Can you work these out from the model? Positions are in its coordinate system, mm. A direction names the side the tool comes from. Round coordinates to 2 decimals unless told otherwise and drop trailing zeros. Loops run counter-clockwise (first coordinate to the right, second up) from the corner with the lowest first, then second, coordinate; pieces in that order, holes last. Notation, with made-up numbers: (60, 49.25) -> (96, 49.25) arc R16 ccw to (96, 53.25) -> close; hole circle Ø6 at (63.5, -26.5). An arc over 180 degrees is marked (long way). Write item = value, one per line.
from build123d import *

# Parameters (mm, degrees)
SKETCH1_R           = 1.6
BOSS_EXTRUDE1_DEPTH = 7.2
SKETCH2_R           = 3.75
CUT_EXTRUDE1_DEPTH  = 5.7
CUT_EXTRUDE2_DEPTH  = 7.5
SKETCH5_W           = 7.75
SKETCH5_H           = 8.9
SKETCH5_W_2         = 9.25
BOSS_EXTRUDE2_DEPTH = 14.4
SKETCH6_W           = 10.1
SKETCH6_H           = 8.4
CUT_EXTRUDE3_DEPTH  = 4.5
FILLET1_R           = 1.75
FILLET2_R           = 1
CHAMFER1_SIZE       = 1.75
CUT_EXTRUDE4_DEPTH  = 3.3
CUT_EXTRUDE5_REACH  = 20.3
SKETCH8_W           = 10.1
SKETCH8_H           = 0.75
SKETCH9_W           = 10.1
SKETCH9_H           = 1.2
BOSS_EXTRUDE3_DEPTH = 5.5


with BuildPart() as part:
    # Sketch1 → Boss-Extrude1 (new body)
    with BuildSketch(Plane.XY):
        with BuildLine():
            ThreePointArc((18.5, 3.75), (22.25, 0), (18.5, -3.75))
            Line((18.5, -3.75), (14.75, -3.75))
            Line((14.75, -3.75), (14.75, -6.5))
            Line((14.75, -6.5), (-14.75, -6.5))
            Line((-14.75, -6.5), (-14.75, -3.75))
            Line((-14.75, -3.75), (-18.5, -3.75))
            ThreePointArc((-18.5, -3.75), (-22.25, 0), (-18.5, 3.75))
            Line((-18.5, 3.75), (-14.75, 3.75))
            Line((-14.75, 3.75), (-14.75, 6.5))
            Line((-14.75, 6.5), (14.75, 6.5))
            Line((14.75, 6.5), (14.75, 3.75))
            Line((14.75, 3.75), (18.5, 3.75))
        make_face()
        with Locations((-18.5, 0)):
            Circle(SKETCH1_R, mode=Mode.SUBTRACT)
        with Locations((18.5, 0)):
            Circle(SKETCH1_R, mode=Mode.SUBTRACT)
    extrude(amount=BOSS_EXTRUDE1_DEPTH)

    # Sketch2 → Cut-Extrude1 (cut)
    with BuildSketch(Plane.XY.offset(7.2)):
        with Locations((-18.5, 0)):
            Circle(SKETCH2_R)
        with Locations((18.5, 0)):
            Circle(SKETCH2_R)
    extrude(amount=-CUT_EXTRUDE1_DEPTH, mode=Mode.SUBTRACT)

    # Sketch4 → Cut-Extrude2 (cut)
    with BuildSketch(Plane.XZ.offset(3.75)):
        Polygon((-18.5, 1.5), (-16.95, 1.5), (-16.95, 3.5), (-14.75, 5.7), (-14.75, 7.2), (-18.5, 7.2), align=None)
        Polygon((18.5, 1.5), (16.95, 1.5), (16.95, 3.5), (14.75, 5.7), (14.75, 7.2), (18.5, 7.2), align=None)
    extrude(amount=-CUT_EXTRUDE2_DEPTH, mode=Mode.SUBTRACT)

    # Sketch5 → Boss-Extrude2 (add)
    with BuildSketch(Plane.XY.offset(7.2)):
        Polygon((-5.8, -5.95), (-14.75, -5.95), (-14.75, 5.95), (-5.8, 5.95), (-5.8, 4.2), (0, 4.2), (4.3, 4.2), (4.3, 5.95), (14.75, 5.95), (14.75, -5.95), (4.3, -5.95), (4.3, -4.2), (0, -4.2), (-5.8, -4.2), align=None)
        with Locations((-10.275, 0)):
            Rectangle(SKETCH5_W, SKETCH5_H, mode=Mode.SUBTRACT)
        with Locations((9.525, 0)):
            Rectangle(SKETCH5_W_2, SKETCH5_H, mode=Mode.SUBTRACT)
    extrude(amount=BOSS_EXTRUDE2_DEPTH)

    # Sketch6 → Cut-Extrude3 (cut)
    with BuildSketch(Plane.XY.offset(21.6)):
        with Locations((-0.75, 0)):
            Rectangle(SKETCH6_W, SKETCH6_H)
    extrude(amount=-CUT_EXTRUDE3_DEPTH, mode=Mode.SUBTRACT)

    # Fillet1
    fillet1_edges = [part.edges().sort_by_distance(p)[0] for p in [
        (4.3, 5.95, 14.4),
        (14.75, 5.95, 14.4),
        (14.75, -5.95, 14.4),
        (4.3, -5.95, 14.4),
        (-5.8, 5.95, 14.4),
        (-14.75, 5.95, 14.4),
        (-14.75, -5.95, 14.4),
        (-5.8, -5.95, 14.4),
    ]]
    fillet(fillet1_edges, radius=FILLET1_R)

    # Fillet2
    fillet2_edges = [part.edges().sort_by_distance(p)[0] for p in [
        (-6.4, 4.45, 14.4),
        (-14.15, 4.45, 14.4),
        (-14.15, -4.45, 14.4),
        (-6.4, -4.45, 14.4),
    ]]
    fillet(fillet2_edges, radius=FILLET2_R)

    # Chamfer1
    chamfer1_edges = [part.edges().sort_by_distance(p)[0] for p in [
        (14.15, 4.45, 14.4),
        (4.9, 4.45, 14.4),
        (4.9, -4.45, 14.4),
        (14.15, -4.45, 14.4),
    ]]
    chamfer(chamfer1_edges, length=CHAMFER1_SIZE)

    # Sketch7 → Cut-Extrude4 (cut)
    with BuildSketch(Plane(origin=(0, 0, 0), x_dir=(-1, 0, 0), z_dir=(0, 0, -1))):
        Polygon((14, -5.75), (14, 5.75), (-14, 5.75), (-14, -5.75), (-5.05, -5.75), (-5.05, -6.5), (5.05, -6.5), (5.05, -5.75), align=None)
    extrude(amount=-CUT_EXTRUDE4_DEPTH, mode=Mode.SUBTRACT)

    # Sketch8 → Cut-Extrude5 (cut, up to next)
    with BuildSketch(Plane(origin=(0, 0, 3.3), x_dir=(-1, 0, 0), z_dir=(0, 0, -1)), mode=Mode.PRIVATE) as cut_extrude5_sk1:
        with Locations((0, -6.125)):
            Rectangle(SKETCH8_W, SKETCH8_H)
    cut_extrude5_tool1 = extrude(cut_extrude5_sk1.sketch, amount=-CUT_EXTRUDE5_REACH, mode=Mode.PRIVATE) & part.part
    add(cut_extrude5_tool1.solids().sort_by_distance((0, -6.125, 3.3))[0], mode=Mode.SUBTRACT)

    # Sketch9 → Boss-Extrude3 (add)
    with BuildSketch(Plane.XZ.offset(5.75)):
        with Locations((0, 3.9)):
            Rectangle(SKETCH9_W, SKETCH9_H)
    extrude(amount=BOSS_EXTRUDE3_DEPTH)


solid = part.part
1. I'm going to push flat-ended pins straight in: pin 1 (6 mm diameter, centred on y = 3.5, z = 5.5, fed in from +X); pin 2 (1.5 mm diameter, centred on x = 11.5, z = 5.5, fed in from -Y); pin 3 (3.5 mm diameter, centred on x = 8, z = 15, fed in from +Y). Where does each tip first touch, or does it pass through?
Entries:
pin_1 = 16.95
pin_2 = -6.5
pin_3 = 5.95
2. We'd pull the mould along X, two halves only. Please class faces 1 (the cylindrical face through (-14.75, -0.06, 3.16)), 2 (the flat face through (-16, -3.75, 2)), 3 (the cylindrical face through (-13.849, 4.165, 14.501)): released by +X, released by -X, zero draft, split by the parting line, or undercut.
Entries:
face_1 = released by -X
face_2 = zero draft
face_3 = undercut
3. Suppose I cut it at A-A, the plane z = 18.5. Count the separate pieces of the cut face and the enclosed holes in it, and give its area (3 significant figures).
Entries:
separate_pieces = 2
enclosed_holes = 2
area = 81.3 mm²
4. For faces 4 (the flat face through (-16, 3.75, 2)), 5 (the flat face through (0, -5.75, 6)), 6 (the flat face through (5.8, -3.6, 14.3)), which set-ups out of +Z, -Z, +X, -X, +Y, -Y let a thin tool reach every point of the face, with its end or its side?
Entries:
face_4 = +Z, -Z, -X, +Y
face_5 = +Z, -Y
face_6 = +Z
5. Suppose I cut it at C-C, the plane z = 2.5. List the corners of the cut face in (x, y) for me.
Entries:
outline = (-16.95, -3.75) -> (-14.75, -3.75) -> (-14.75, -6.5) -> (-5.05, -6.5) -> (-5.05, -5.75) -> (-14, -5.75) -> (-14, 5.75) -> (14, 5.75) -> (14, -5.75) -> (5.05, -5.75) -> (5.05, -6.5) -> (14.75, -6.5) -> (14.75, -3.75) -> (16.95, -3.75) -> (16.95, -3.41) arc R3.75 cw to (16.95, 3.41) -> (16.95, 3.75) -> (14.75, 3.75) -> (14.75, 6.5) -> (-14.75, 6.5) -> (-14.75, 3.75) -> (-16.95, 3.75) -> (-16.95, 3.41) arc R3.75 cw to (-16.95, -3.41) -> close
6. I need wall thicknesses on line 1 (X direction, y = 0, z = 0.9); line 2 (X direction, y = -2.25, z = 19.5); line 3 (Y direction, x = 18.5, z = 1.05). Which ranges of each line are inside material? Lowest first, please. Write a range as [from, to].
Entries:
line_1 = [-22.25, -20.1], [-16.9, -14], [14, 16.9], [20.1, 22.25]
line_2 = [-14.75, -14.15], [-6.4, -5.8], [4.3, 4.9], [14.15, 14.75]
line_3 = [-3.75, -1.6], [1.6, 3.75]
7. Suppose I cut it at B-B, the plane x = 9. List the corners of the cut face in (y, z) for me.
Entries:
outline = (-6.5, 0) -> (-5.75, 0) -> (-5.75, 3.3) -> (5.75, 3.3) -> (5.75, 0) -> (6.5, 0) -> (6.5, 7.2) -> (5.95, 7.2) -> (5.95, 21.6) -> (4.45, 21.6) -> (4.45, 7.2) -> (-4.45, 7.2) -> (-4.45, 21.6) -> (-5.95, 21.6) -> (-5.95, 7.2) -> (-6.5, 7.2) -> close
